Here's how the part is built. I have some questions about the finished solid (model axes, mm). Round coordinates to 2 decimals unless told otherwise and drop trailing zeros. Loops run counter-clockwise (first coordinate to the right, second up) from the corner with the lowest first, then second, coordinate; pieces in that order, holes last. Notation, with made-up numbers: (-13, -25.75) -> (-6, -25.75) arc R14 cw to (-6, -3.75) -> close; hole circle Ø8 at (23, 1.25). An arc over 180 degrees is marked (long way). One line per item, written item: value. Start each with the question number.
```python
from build123d import *

# Parameters (mm, degrees)
SKETCH1_W                                      = 12.7
SKETCH1_H                                      = 9.525
BOSS_EXTRUDE1_DEPTH                            = 419.1
CBORE_FOR_8_SOCKET_HEAD_CAP_SCREW1_D           = 4.9149
CBORE_FOR_8_SOCKET_HEAD_CAP_SCREW1_CBORE_D     = 7.9375
CBORE_FOR_8_SOCKET_HEAD_CAP_SCREW1_CBORE_DEPTH = 4.1656


with BuildPart() as part:
    # Sketch1 → Boss-Extrude1 (new body)
    with BuildSketch(Plane(origin=(0, 0, 0), x_dir=(1, 0, 0), z_dir=(0, 1, 0))):
        with Locations((-0.36888069, 2.767280084)):
            Rectangle(SKETCH1_W, SKETCH1_H)
    extrude(amount=BOSS_EXTRUDE1_DEPTH)

    # CBORE for #8 Socket Head Cap Screw1 (through all)
    with Locations(Plane(origin=(0, 0, -7.529780084), x_dir=(-1, 0, 0), z_dir=(0, 0, -1))):
        with Locations((0.36888069, 414.3375), (0.36888069, 4.7625)):
            CounterBoreHole(CBORE_FOR_8_SOCKET_HEAD_CAP_SCREW1_D / 2, CBORE_FOR_8_SOCKET_HEAD_CAP_SCREW1_CBORE_D / 2, CBORE_FOR_8_SOCKET_HEAD_CAP_SCREW1_CBORE_DEPTH)


solid = part.part
```
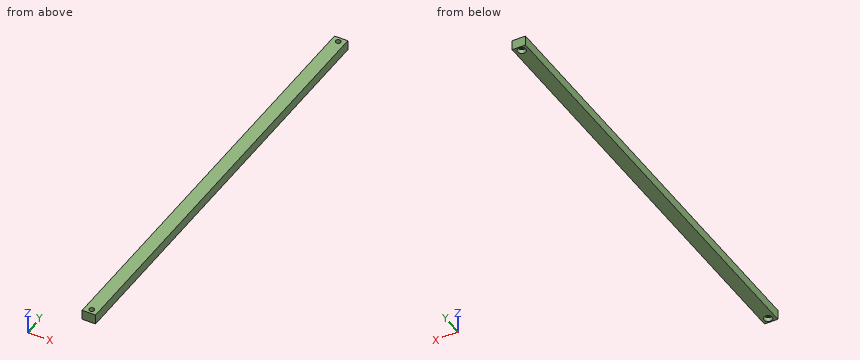
Q1. I want a section at B-B on z = -6. Please give me the cut outline in (x, y).
Q2. If I drill on line 1 along Y through (x, z) = (-1, -0.75); line 2 along Y through (x, z) = (0, -7), over which ranges is the centre line in solid material (lowest first)?
Q3. I want a section at A-A on x = 0. Please give me the cut outline in (y, z), plus the area to 3 significant figures.
Q4. Will these pins go through, and if not, where does the flat tip stop? P1, Ø7, axis at x = -0.37, y = 4.76, coming from the -Z side; P2, Ø1.5, axis at x = -1.5, z = 0.5, coming from the -Y side.
Answers below:
1. outline: (-6.72, 0) -> (5.98, 0) -> (5.98, 419.1) -> (-6.72, 419.1) -> close; hole circle Ø7.94 at (-0.37, 4.76); hole circle Ø7.94 at (-0.37, 414.34)
2. line 1: y = 0 to 2.39, 7.14 to 411.96, 416.71 to 419.1
2. line 2: y = 0 to 0.81, 8.71 to 410.39, 418.29 to 419.1
3. outline: (0, -7.53) -> (0.81, -7.53) -> (0.81, -3.36) -> (2.33, -3.36) -> (2.33, 2) -> (0, 2) -> close; (7.19, -3.36) -> (8.71, -3.36) -> (8.71, -7.53) -> (410.39, -7.53) -> (410.39, -3.36) -> (411.91, -3.36) -> (411.91, 2) -> (7.19, 2) -> close; (416.77, -3.36) -> (418.29, -3.36) -> (418.29, -7.53) -> (419.1, -7.53) -> (419.1, 2) -> (416.77, 2) -> close
3. area: 3,870 mm^2
4. P1: stops at z = -3.36
4. P2: stops at y = 0
